Read the model definition and answer for the solid it produces. Units are mm, in the model's axes. A direction names the side the tool comes from. Coordinates: 2 decimals unless noted, no trailing zeros. Loops run counter-clockwise (first coordinate to the right, second up) from the corner with the lowest first, then second, coordinate; pieces in that order, holes last.
Q1. Section A-A (y = 9) is taken. Give the vertices of the cut face in (x, z), then the cut area to 3 significant figures.
Q2. The mould has two halves that part along Y. Classify faces 1 (the face through (53, 0, -27)), 2 (the face through (41.229, 24.496, -19.713)), 3 (the face through (36.455, 20.89, -25.568)): pulls with the +Y half, pulls with the -Y half, needs draft (parallel to the pull), parting line crosses it, or undercut.
Q3. Which of the six approach directions +Z, -Z, +X, -X, +Y, -Y give full straight-line access (tool end or side, diameter ignored) to faces 4 (the face through (47.786, 21.14, -27.987)), 5 (the face through (43, 24.5, -33.7))?
Q4. Section B-B (y = 15.5) is taken. Give the vertices of the cut face in (x, z).
Q5. Straight lines are drawn through the part: line 1 (Z direction, x = 49.75, y = 22); line 2 (Y direction, x = 53.25, z = -28); line 3 (X direction, y = 1.75, z = -26.25). For each, find the intervals that lie inside material, in ascending order.
Q6. Flat-ended cylindrical pins translate along their axes: P1, Ø3, axis at y = 18.5, z = -31.5, coming from the +X side; P2, Ø3, axis at y = 6.5, z = -32.5, coming from the +X side; P3, Ø8, axis at y = 6, z = -30, coming from the -X side. Find the tip coordinate at first contact, or state that the pin passes through.
from build123d import *

# Parameters (mm, degrees)
BOSS_EXTRUDE2_DEPTH             = 26
CUT_EXTRUDE7_DEPTH              = 71.182431461
CUT_EXTRUDE8_DEPTH              = 59.485252348
FILLET6_R                       = 5
M5_TAPPED_HOLE1_D               = 4.2
M5_TAPPED_HOLE1_DEPTH           = 4.7381927
M5_TAPPED_HOLE1_TIP             = 1.2618073
M5_TAPPED_HOLE1_ON_FACE_2_D     = 4.2
M5_TAPPED_HOLE1_ON_FACE_2_DEPTH = 4.7381927
M5_TAPPED_HOLE1_ON_FACE_2_TIP   = 1.2618073


with BuildPart() as part:
    # 草图1 → Boss-Extrude2 (new body)
    with BuildSketch(Plane(origin=(0, 0, 0), x_dir=(1, 0, 0), z_dir=(0, 1, 0))):
        Polygon((29.300589914, 18.286975519), (51.945589914, 18.286975519), (54.914973752, 35.127188096), (32.269973752, 35.127188096), align=None)
        Polygon((29.300589914, 18.286975519), (51.945589914, 18.286975519), (51.262759613, 14.414452446), align=None)
    extrude(amount=BOSS_EXTRUDE2_DEPTH)

    # Sketch3 → Cut-Extrude7 (cut, through all)
    with BuildSketch(Plane(origin=(0, 26, 0), x_dir=(1, 0, 0), z_dir=(0, 1, 0))):
        Polygon((29.300589914, 18.286975519), (51.945589914, 18.286975519), (51.262759613, 14.414452446), align=None)
    extrude(amount=-CUT_EXTRUDE7_DEPTH, mode=Mode.SUBTRACT)

    # Sketch2 → Cut-Extrude8 (cut, through all)
    with BuildSketch(Plane(origin=(4.010777888, 0, -22.746251717), x_dir=(0.984807753012208, 0, 0.17364817766693091), z_dir=(-0.17364817766693091, 0, 0.984807753012208))):
        with BuildLine():
            Line((27.330433925, 0), (46.330433925, 0))
            ThreePointArc((46.330433925, 0), (36.830433925, 9.5), (27.330433925, 0))
        make_face()
    extrude(amount=-CUT_EXTRUDE8_DEPTH, mode=Mode.SUBTRACT)

    # Fillet6
    fillet6_edges = [part.edges().sort_by_distance(p)[0] for p in [
        (40.623089914, 26, -18.286975519),
        (43.592473752, 26, -35.127188096),
    ]]
    fillet(fillet6_edges, radius=FILLET6_R)

    # M5 Tapped Hole1
    with Locations(Plane(origin=(53.537445864, 21, -27.314839229), x_dir=(-0.173648177667, 0, 0.984807753012), z_dir=(0.984807753012, 0, 0.173648177667))):
        with Locations((0, 0)):
            Hole(M5_TAPPED_HOLE1_D / 2, depth=M5_TAPPED_HOLE1_DEPTH)
            with Locations((0, 0, -(M5_TAPPED_HOLE1_DEPTH + M5_TAPPED_HOLE1_TIP / 2))):  # 118° drill point
                Cone(0, M5_TAPPED_HOLE1_D / 2, M5_TAPPED_HOLE1_TIP, mode=Mode.SUBTRACT)

    # M5 Tapped Hole1 on face 2
    with Locations(Plane(origin=(30.701085573, 21, -26.229581085), x_dir=(0.17364796312, 0, -0.984807790843), z_dir=(-0.984807790843, 0, -0.17364796312))):
        with Locations((0, 0)):
            Hole(M5_TAPPED_HOLE1_ON_FACE_2_D / 2, depth=M5_TAPPED_HOLE1_ON_FACE_2_DEPTH)
            with Locations((0, 0, -(M5_TAPPED_HOLE1_ON_FACE_2_DEPTH + M5_TAPPED_HOLE1_ON_FACE_2_TIP / 2))):  # 118° drill point
                Cone(0, M5_TAPPED_HOLE1_ON_FACE_2_D / 2, M5_TAPPED_HOLE1_ON_FACE_2_TIP, mode=Mode.SUBTRACT)


solid = part.part
Numbers:
1. outline: (29.3, -18.29) - (32.27, -35.13) - (40.5, -35.13) - (37.53, -18.29) - close; (43.71, -18.29) - (46.68, -35.13) - (54.91, -35.13) - (51.95, -18.29) - close
1. area: 277 mm2
2. face 1: pulls with the -Y half
2. face 2: pulls with the +Y half
2. face 3: undercut
3. face 4: none
3. face 5: -Z, +X, -X, +Y
4. outline: (29.3, -18.29) - (32.27, -35.13) - (54.91, -35.13) - (51.95, -18.29) - close
5. line 1: z = -35.03 to -29.86, -26.11 to -18.39
5. line 2: y = 0 to 19, 23 to 26
5. line 3: x = 30.7 to 32.55, 51.51 to 53.35
6. P1: stops at x = 54.54
6. P2: stops at x = 54.72
6. P3: stops at x = 30.66
